Can you work these out from the model? Positions are in its coordinate system, mm. Face numbers are marked on the shaded views. A direction names the side the tool comes from. Round coordinates to 2 decimals unless told otherwise and drop trailing zeros. Order: outer loops, then holes, each group sorted by start corner. A loop starts at its lowest first (then second) coordinate and runs counter-clockwise, first axis right, second up. Notation, with made-up numbers: (83, 33) -> (97, 33) arc R18 cw to (97, 54) -> close; hole circle Ø9 at (-29.75, 86.5). An arc over 180 degrees is marked (long way). One line per item, written item: value.
```python
from build123d import *

# Parameters (mm, degrees)
BOSS_EXTRUDE1_DEPTH = 139.7
CUT_EXTRUDE1_DEPTH  = 3.175
SKETCH5_W           = 3.175
SKETCH5_H           = 12.7
BOSS_EXTRUDE2_DEPTH = 3.175
SKETCH8_R           = 1.27
CUT_EXTRUDE2_DEPTH  = 3.175


with BuildPart() as part:
    # Sketch1 → Boss-Extrude1 (new body)
    with BuildSketch(Plane(origin=(0, 0, 0), x_dir=(0, 0, -1), z_dir=(1, 0, 0))):
        with BuildLine():
            Line((-118.11, -50.8), (-106.68, -47.625))
            Line((-106.68, -47.625), (-47.625, -47.625))
            ThreePointArc((-47.625, -47.625), (-13.949039546, -33.675960454), (0, 0))
            Line((0, 0), (0, 254))
            Line((0, 254), (3.175, 254))
            Line((3.175, 254), (3.175, 0))
            ThreePointArc((3.175, 0), (-11.703975516, -35.921024484), (-47.625, -50.8))
            Line((-47.625, -50.8), (-118.11, -50.8))
        make_face()
    extrude(amount=BOSS_EXTRUDE1_DEPTH)

    # Sketch4 → Cut-Extrude1 (cut, symmetric)
    with BuildSketch(Plane.XY):
        Polygon((0, 204.6605), (0, 201.7395), (6.35, 201.7395), (6.35, 200.025), (8.73125, 200.025), (8.73125, 201.7395), (12.7, 201.7395), (12.7, 203.2), (12.7, 204.6605), (8.73125, 204.6605), (8.73125, 206.375), (6.35, 206.375), (6.35, 204.6605), align=None)
        Polygon((0, 153.8605), (0, 150.9395), (6.35, 150.9395), (6.35, 149.225), (8.73125, 149.225), (8.73125, 150.9395), (12.7, 150.9395), (12.7, 152.4), (12.7, 153.8605), (8.73125, 153.8605), (8.73125, 155.575), (6.35, 155.575), (6.35, 153.8605), align=None)
        Polygon((0, 103.0605), (0, 100.1395), (6.35, 100.1395), (6.35, 98.425), (8.73125, 98.425), (8.73125, 100.1395), (12.7, 100.1395), (12.7, 101.6), (12.7, 103.0605), (8.73125, 103.0605), (8.73125, 104.775), (6.35, 104.775), (6.35, 103.0605), align=None)
        Polygon((0, 52.2605), (0, 49.3395), (6.35, 49.3395), (6.35, 47.625), (8.73125, 47.625), (8.73125, 49.3395), (12.7, 49.3395), (12.7, 50.8), (12.7, 52.2605), (8.73125, 52.2605), (8.73125, 53.975), (6.35, 53.975), (6.35, 52.2605), align=None)
        Polygon((0, 1.4605), (0, -1.4605), (6.35, -1.4605), (6.35, -3.175), (8.73125, -3.175), (8.73125, -1.4605), (12.7, -1.4605), (12.7, 0), (12.7, 1.4605), (8.73125, 1.4605), (8.73125, 3.175), (6.35, 3.175), (6.35, 1.4605), align=None)
    cut_extrude1 = extrude(amount=CUT_EXTRUDE1_DEPTH, both=True, mode=Mode.SUBTRACT)

    # Sketch5 → Boss-Extrude2 (add)
    with BuildSketch(Plane.XY):
        with Locations((-1.5875, 228.6)):
            Rectangle(SKETCH5_W, SKETCH5_H)
        with Locations((-1.5875, 177.8)):
            Rectangle(SKETCH5_W, SKETCH5_H)
        with Locations((-1.5875, 25.4)):
            Rectangle(SKETCH5_W, SKETCH5_H)
        with Locations((-1.5875, 76.085444403)):
            Rectangle(SKETCH5_W, SKETCH5_H)
        with Locations((-1.5875, 127.114555597)):
            Rectangle(SKETCH5_W, SKETCH5_H)
    boss_extrude2 = extrude(amount=-BOSS_EXTRUDE2_DEPTH)

    # Mirror1: Cut-Extrude1, Boss-Extrude2 across plane
    add(cut_extrude1.mirror(Plane(origin=(69.85, 0, 0), x_dir=(0, 0, 1), z_dir=(1, 0, 0))), mode=Mode.SUBTRACT)
    add(boss_extrude2.mirror(Plane(origin=(69.85, 0, 0), x_dir=(0, 0, 1), z_dir=(1, 0, 0))))

    # Sketch8 → Cut-Extrude2 (cut)
    with BuildSketch(Plane(origin=(0, -47.625, 0), x_dir=(1, 0, 0), z_dir=(0, 1, 0))):
        with Locations(Location((2.54, -51.054, 0), (0, 0, 270))):
            Circle(SKETCH8_R)
        with Locations(Location((2.54, -76.454, 0), (0, 0, 270))):
            Circle(SKETCH8_R)
        with Locations(Location((2.54, -101.854, 0), (0, 0, 270))):
            Circle(SKETCH8_R)
    cut_extrude2 = extrude(amount=-CUT_EXTRUDE2_DEPTH, mode=Mode.SUBTRACT)

    # Mirror2: Cut-Extrude2 across plane
    add(cut_extrude2.mirror(Plane(origin=(69.85, 0, 0), x_dir=(0, 0, 1), z_dir=(1, 0, 0))), mode=Mode.SUBTRACT)


solid = part.part
```
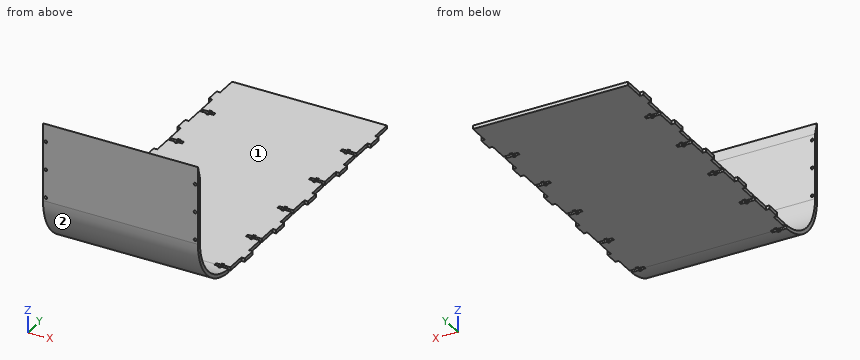
Q1. Please list where these lines run through material, in increasing order: line 1 along Y through (x, z) = (67, 46.5); line 2 along Z through (x, y) = (60.5, 187.5) (3 decimals); line 3 along Y through (x, z) = (19.5, 9).
Answers below:
line 1: -50.79 to -47.61
line 2: -3.175 to 0
line 3: -33 to -27.86
Q2. Will these pins go through, and if not, where does the flat tip stop? pin 1 Ø1 at (x, y) = (39.5, 38) entering from +Z; pin 2 Ø3.5 at (x, z) = (10.5, -1) entering from -Y; pin 3 Ø0.9 at (y, z) = (155, -2) entering from +X.
Answers below:
pin 1: z = 0
pin 2: y = -19.58
pin 3: x = 139.7
Q3. I want a section at B-B on z = 91. List the corners of the cut face in (x, y) for me (3 decimals), plus the area to 3 significant figures.
Answers below:
outline: (0, -50.8) -> (139.7, -50.8) -> (139.7, -47.625) -> (0, -47.625) -> close
area: 444 mm^2
Q4. I want a section at A-A on x = 55.5. List the corners of the cut face in (y, z) for me (3 decimals), plus the area to 3 significant figures.
Answers below:
outline: (-50.8, 47.625) arc R50.8 ccw to (0, -3.175) -> (254, -3.175) -> (254, 0) -> (0, 0) arc R47.625 cw to (-47.625, 47.625) -> (-47.625, 106.68) -> (-50.8, 118.11) -> close
area: 1,260 mm^2
Q5. On a 3-axis mill with a long thin cutter (end or side, diameter ignored), from which of +Z, -Z, +X, -X, +Y, -Y can I reach the whole of each face in a straight line? I mean the marked faces 1 and 2. Say none if no direction works.
Answers below:
face 1: +Z, +X, -X, +Y
face 2: -Z, +X, -X, -Y
Q6. I want a section at C-C on y = 229.5. List the corners of the cut face in (x, z) for me (3 decimals).
Answers below:
outline: (-3.175, -3.175) -> (142.875, -3.175) -> (142.875, 0) -> (-3.175, 0) -> close
